```python
from build123d import *

# Parameters (mm, degrees)
SKETCH1_W           = 55
SKETCH1_H           = 20
SKETCH1_R           = 2.279195974
BOSS_EXTRUDE1_DEPTH = 10
BOSS_EXTRUDE1_DRAFT = 2
FILLET1_R           = 2
FILLET2_R           = 2


with BuildPart() as part:
    # Sketch1 → Boss-Extrude1 (with draft: the straight prism first)
    with BuildSketch(Plane.XY):
        with Locations((-40.5, 12.750475985)):
            Rectangle(SKETCH1_W, SKETCH1_H)
        with Locations((-22.9997867, 12.458174308)):
            Circle(SKETCH1_R, mode=Mode.SUBTRACT)
    extrude(amount=BOSS_EXTRUDE1_DEPTH)
    # Boss-Extrude1: the draft: its side faces are tilted about the plane it starts from
    boss_extrude1_sides = [part.faces().sort_by_distance(p)[0] for p in [
        (-13, 12.750475985, 5),
        (-40.5, 22.750475985, 5),
        (-68, 12.750475985, 5),
        (-40.5, 2.750475985, 5),
        (-25.278982673, 12.458174308, 5),
    ]]
    draft(boss_extrude1_sides, Plane.XY, BOSS_EXTRUDE1_DRAFT)

    # Fillet1
    fillet1_edges = [part.edges().sort_by_distance(p)[0] for p in [
        (-67.650792305, 12.750475985, 10),
        (-40.5, 3.09968368, 10),
        (-13.349207695, 12.750475985, 10),
        (-40.5, 22.40126829, 10),
    ]]
    fillet(fillet1_edges, radius=FILLET1_R)

    # Fillet2
    # the kernel refuses this fillet: 2 mm, written as the material it takes off along each edge
    with BuildSketch(Plane(origin=(-65.719414755, 20.469890741, 8), x_dir=(-0.719128245661317, 0.024250870657585206, -0.6944540744818377), z_dir=(-0.5638062984383352, 0.5638062984383351, 0.6035270629247093))) as fillet2_piece_1_section:
        Polygon((-4.062392326, -4.062392326), (4.062392326, -4.062392326), (4.062392326, 4.062392326), (-4.062392326, 4.062392326), align=None)
    fillet2_piece_1 = extrude(amount=4.062392326, mode=Mode.PRIVATE)
    fillet2_piece_1 = split(fillet2_piece_1, bisect_by=Plane(origin=(-65.719414755, 20.469890741, 8), z_dir=(0.03487826274237467, -0.03487826274237466, 0.9987827659587183)), keep=Keep.TOP, mode=Mode.PRIVATE)
    fillet2_piece_1 = split(fillet2_piece_1, bisect_by=Plane(origin=(-65.719414755, 20.469890741, 8), z_dir=(0, 1, 0)), keep=Keep.TOP, mode=Mode.PRIVATE)
    fillet2_piece_1 = split(fillet2_piece_1, bisect_by=Plane(origin=(-65.719414755, 20.469890741, 8), z_dir=(-1, 0, 0)), keep=Keep.TOP, mode=Mode.PRIVATE)
    fillet2_piece_1 = split(fillet2_piece_1, bisect_by=Plane(origin=(-65.719414755, 22.468672395, 8.069798993), z_dir=(0, -0.9993908270190958, -0.03489949670250102)), keep=Keep.TOP, mode=Mode.PRIVATE)
    fillet2_piece_1 = split(fillet2_piece_1, bisect_by=Plane(origin=(-67.71819641, 20.469890741, 8.069798993), z_dir=(0.9993908270190958, 0, -0.03489949670250102)), keep=Keep.TOP, mode=Mode.PRIVATE)
    fillet2_piece_1 = split(fillet2_piece_1, bisect_by=Plane(origin=(-65.719414755, 20.469890741, 10), z_dir=(0, 0, -1)), keep=Keep.TOP, mode=Mode.PRIVATE)
    fillet2_piece_1 = fillet2_piece_1 - Plane(origin=(-65.719414755, 20.469890741, 8), x_dir=(0.5638062984383352, -0.5638062984383351, -0.6035270629247093), z_dir=(-0.719128245661317, 0.024250870657585206, -0.6944540744818377)) * Sphere(FILLET2_R, mode=Mode.PRIVATE)
    add(fillet2_piece_1, mode=Mode.SUBTRACT)
    with BuildSketch(Plane(origin=(-15.280585245, 20.469890741, 8), x_dir=(0.024250870657585296, 0.719128245661317, -0.6944540744818377), z_dir=(0.5638062984383351, 0.5638062984383351, 0.6035270629247093))) as fillet2_piece_2_section:
        Polygon((-4.062392326, -4.062392326), (4.062392326, -4.062392326), (4.062392326, 4.062392326), (-4.062392326, 4.062392326), align=None)
    fillet2_piece_2 = extrude(amount=4.062392326, mode=Mode.PRIVATE)
    fillet2_piece_2 = split(fillet2_piece_2, bisect_by=Plane(origin=(-15.280585245, 20.469890741, 8), z_dir=(-0.03487826274237467, -0.034878262742374676, 0.9987827659587183)), keep=Keep.TOP, mode=Mode.PRIVATE)
    fillet2_piece_2 = split(fillet2_piece_2, bisect_by=Plane(origin=(-15.280585245, 20.469890741, 8), z_dir=(1, 0, 0)), keep=Keep.TOP, mode=Mode.PRIVATE)
    fillet2_piece_2 = split(fillet2_piece_2, bisect_by=Plane(origin=(-15.280585245, 20.469890741, 8), z_dir=(0, 1, 0)), keep=Keep.TOP, mode=Mode.PRIVATE)
    fillet2_piece_2 = split(fillet2_piece_2, bisect_by=Plane(origin=(-13.28180359, 20.469890741, 8.069798993), z_dir=(-0.9993908270190958, 0, -0.03489949670250102)), keep=Keep.TOP, mode=Mode.PRIVATE)
    fillet2_piece_2 = split(fillet2_piece_2, bisect_by=Plane(origin=(-15.280585245, 22.468672395, 8.069798993), z_dir=(0, -0.9993908270190958, -0.03489949670250102)), keep=Keep.TOP, mode=Mode.PRIVATE)
    fillet2_piece_2 = split(fillet2_piece_2, bisect_by=Plane(origin=(-15.280585245, 20.469890741, 10), z_dir=(0, 0, -1)), keep=Keep.TOP, mode=Mode.PRIVATE)
    fillet2_piece_2 = fillet2_piece_2 - Plane(origin=(-15.280585245, 20.469890741, 8), x_dir=(-0.5638062984383351, -0.5638062984383351, -0.6035270629247093), z_dir=(0.024250870657585296, 0.719128245661317, -0.6944540744818377)) * Sphere(FILLET2_R, mode=Mode.PRIVATE)
    add(fillet2_piece_2, mode=Mode.SUBTRACT)
    with BuildSketch(Plane(origin=(-65.719414755, 5.03106123, 8), x_dir=(0.7191282456613168, 0.0242508706575854, 0.6944540744818378), z_dir=(-0.5638062984383351, -0.5638062984383351, 0.6035270629247093))) as fillet2_piece_3_section:
        Polygon((-4.062392326, -4.062392326), (4.062392326, -4.062392326), (4.062392326, 4.062392326), (-4.062392326, 4.062392326), align=None)
    fillet2_piece_3 = extrude(amount=4.062392326, mode=Mode.PRIVATE)
    fillet2_piece_3 = split(fillet2_piece_3, bisect_by=Plane(origin=(-65.719414755, 5.03106123, 8), z_dir=(0.03487826274237467, 0.034878262742374676, 0.9987827659587183)), keep=Keep.TOP, mode=Mode.PRIVATE)
    fillet2_piece_3 = split(fillet2_piece_3, bisect_by=Plane(origin=(-65.719414755, 5.03106123, 8), z_dir=(0, -1, 0)), keep=Keep.TOP, mode=Mode.PRIVATE)
    fillet2_piece_3 = split(fillet2_piece_3, bisect_by=Plane(origin=(-65.719414755, 5.03106123, 8), z_dir=(-1, 0, 0)), keep=Keep.TOP, mode=Mode.PRIVATE)
    fillet2_piece_3 = split(fillet2_piece_3, bisect_by=Plane(origin=(-65.719414755, 3.032279576, 8.069798993), z_dir=(0, 0.9993908270190958, -0.03489949670250102)), keep=Keep.TOP, mode=Mode.PRIVATE)
    fillet2_piece_3 = split(fillet2_piece_3, bisect_by=Plane(origin=(-67.71819641, 5.03106123, 8.069798993), z_dir=(0.9993908270190958, 0, -0.03489949670250102)), keep=Keep.TOP, mode=Mode.PRIVATE)
    fillet2_piece_3 = split(fillet2_piece_3, bisect_by=Plane(origin=(-65.719414755, 5.03106123, 10), z_dir=(0, 0, -1)), keep=Keep.TOP, mode=Mode.PRIVATE)
    fillet2_piece_3 = fillet2_piece_3 - Plane(origin=(-65.719414755, 5.03106123, 8), x_dir=(0.5638062984383351, 0.5638062984383351, -0.6035270629247093), z_dir=(0.7191282456613168, 0.0242508706575854, 0.6944540744818378)) * Sphere(FILLET2_R, mode=Mode.PRIVATE)
    add(fillet2_piece_3, mode=Mode.SUBTRACT)
    with BuildSketch(Plane(origin=(-15.280585245, 5.03106123, 8), x_dir=(-0.024250870657585296, 0.719128245661317, 0.6944540744818377), z_dir=(0.5638062984383352, -0.5638062984383351, 0.6035270629247093))) as fillet2_piece_4_section:
        Polygon((-4.062392326, -4.062392326), (4.062392326, -4.062392326), (4.062392326, 4.062392326), (-4.062392326, 4.062392326), align=None)
    fillet2_piece_4 = extrude(amount=4.062392326, mode=Mode.PRIVATE)
    fillet2_piece_4 = split(fillet2_piece_4, bisect_by=Plane(origin=(-15.280585245, 5.03106123, 8), z_dir=(-0.03487826274237467, 0.03487826274237466, 0.9987827659587183)), keep=Keep.TOP, mode=Mode.PRIVATE)
    fillet2_piece_4 = split(fillet2_piece_4, bisect_by=Plane(origin=(-15.280585245, 5.03106123, 8), z_dir=(1, 0, 0)), keep=Keep.TOP, mode=Mode.PRIVATE)
    fillet2_piece_4 = split(fillet2_piece_4, bisect_by=Plane(origin=(-15.280585245, 5.03106123, 8), z_dir=(0, -1, 0)), keep=Keep.TOP, mode=Mode.PRIVATE)
    fillet2_piece_4 = split(fillet2_piece_4, bisect_by=Plane(origin=(-13.28180359, 5.03106123, 8.069798993), z_dir=(-0.9993908270190958, 0, -0.03489949670250102)), keep=Keep.TOP, mode=Mode.PRIVATE)
    fillet2_piece_4 = split(fillet2_piece_4, bisect_by=Plane(origin=(-15.280585245, 3.032279576, 8.069798993), z_dir=(0, 0.9993908270190958, -0.03489949670250102)), keep=Keep.TOP, mode=Mode.PRIVATE)
    fillet2_piece_4 = split(fillet2_piece_4, bisect_by=Plane(origin=(-15.280585245, 5.03106123, 10), z_dir=(0, 0, -1)), keep=Keep.TOP, mode=Mode.PRIVATE)
    fillet2_piece_4 = fillet2_piece_4 - Plane(origin=(-15.280585245, 5.03106123, 8), x_dir=(-0.5638062984383352, 0.5638062984383351, -0.6035270629247093), z_dir=(-0.024250870657585296, 0.719128245661317, 0.6944540744818377)) * Sphere(FILLET2_R, mode=Mode.PRIVATE)
    add(fillet2_piece_4, mode=Mode.SUBTRACT)
    with BuildSketch(Plane(origin=(-12.825820961, 2.576296946, -4.987835068), x_dir=(0.0012172338155652697, 0.9993915682994698, -0.034857015847091166), z_dir=(-0.03487826274237467, 0.03487826274237466, 0.9987827659587183)), Plane(origin=(-68.174179039, 2.576296946, -4.987835068), x_dir=(0.99939156829947, -0.0012172338155659363, -0.034857015847091145), z_dir=(0.03487826274237467, 0.034878262742374676, 0.9987827659587183))) as fillet2_piece_5:
        with BuildLine():
            CenterArc((FILLET2_R * 0.998782765959, FILLET2_R), FILLET2_R, 180.069784837, 89.930215163)
            Line((-FILLET2_R * 0.00121649230961, FILLET2_R * 0.99878202513), (0, 0))
            Line((0, 0), (FILLET2_R * 0.998782765959, 0))
        make_face()
    extrude(amount=13.14326166, mode=Mode.SUBTRACT)
    with BuildSketch(Plane(origin=(-68.174179039, 22.924655024, -4.987835068), x_dir=(0.99939156829947, 0.001217233815566174, -0.03485701584709114), z_dir=(0.03487826274237467, -0.03487826274237466, 0.9987827659587183)), Plane(origin=(-12.825820961, 22.924655024, -4.987835068), x_dir=(0.0012172338155670467, -0.9993915682994698, -0.03485701584709112), z_dir=(-0.03487826274237467, -0.034878262742374676, 0.9987827659587183))) as fillet2_piece_6:
        with BuildLine():
            CenterArc((FILLET2_R * 0.998782765959, -FILLET2_R), FILLET2_R, 90, 89.930215163)
            Line((-FILLET2_R * 0.00121649230961, -FILLET2_R * 0.99878202513), (0, 0))
            Line((0, 0), (FILLET2_R * 0.998782765959, 0))
        make_face()
    extrude(amount=13.14326166, mode=Mode.SUBTRACT)


solid = part.part
```
CAD build for the part. Positions are in the model's coordinates, mm. Give positions to 0.01 mm unless a question says otherwise; leave off trailing zeros. Write each loop counter-clockwise with the first axis right and the second up, starting at its lowest first coordinate (ties: lowest second). Pieces come first, ordered by that corner, then holes. Notation, with made-up numbers: M -40,89 L -7,89 A28 ccw -7,127 Z; hole C 78.5,15 d4. An arc over 180 degrees is marked long. Return JSON: item names as keys, results as strings. Group by question number.
(1) Band-saw the part on A-A (x = -31.5). Give the cut face in (y, z).
(2) Mould opens along X. For faces 1 (the face through (-13.7, 22, 4)), 2 (the face through (-67.3, 22, 4)), 3 (the face through (-23.32, 14.89, 4.93)) say: pulls with the +X half, pulls with the -X half, needs draft (parallel to the pull), parting line crosses it, or undercut.
(3) Flat gauge pins, fed straight in: pin 1 Ø4 at (y, z) = (14, 8.5) entering from +X; pin 2 Ø2 at (y, z) = (8.5, 4.5) entering from -X. Where does each tip first touch, or does it go through?
(4) Drill centre lines: L1, parallel to Y at x = -27, z = 8; L2, parallel to Y at x = -23, z = 4.75; L3, parallel to X at y = 12.5, z = 7.5. Where is each one in solid material? Low to high. Write a range as [from, to].
Entries:
{
 "1": {"outline": "M 2.75,0 L 22.75,0 L 22.47,8.07 A2 ccw 20.47,10 L 5.03,10 A2 ccw 3.03,8.07 Z"},
 "2": {"face 1": "pulls with the +X half", "face 2": "pulls with the -X half", "face 3": "undercut"},
 "3": {"pin 1": "stops at x = -13.23", "pin 2": "stops at x = -67.88"},
 "4": {"L1": "y = [3.03, 22.47]", "L2": "y = [2.92, 10.01], [14.9, 22.58]", "L3": "x = [-67.74, -25.54], [-20.46, -13.26]"}
}
